Check sheet for the modelled part. Datum: model origin and axes. Units: mm. A direction names the side the tool comes from. Round coordinates to 2 decimals unless told otherwise and drop trailing zeros. Order: outer loops, then holes, each group sorted by start corner. A loop starts at its lowest first (then second) coordinate and runs counter-clockwise, first axis right, second up. Notation, with made-up numbers: (-8.75, 43.25) -> (2.25, 43.25) arc R20 cw to (2.25, 62.25) -> close; hole circle Ø8 at (26.5, -15.5). An arc over 180 degrees is marked (long way). Answer in a Markdown table with one row per item.
```python
from build123d import *

# Parameters (mm, degrees)
SKETCH1_W           = 42
SKETCH1_H           = 42
BOSS_EXTRUDE1_DEPTH = 10.95
CUT_EXTRUDE1_REACH  = 38.9
FILLET1_R           = 2
CUT_EXTRUDE2_DEPTH  = 21.9


with BuildPart() as part:
    # Sketch1 → Boss-Extrude1 (new, symmetric)
    with BuildSketch(Plane.XY):
        Rectangle(SKETCH1_W, SKETCH1_H)
    extrude(amount=BOSS_EXTRUDE1_DEPTH, both=True)

    # Sketch2 → Cut-Extrude1 (cut, up to next)
    with BuildSketch(Plane.XY.offset(10.95), mode=Mode.PRIVATE) as cut_extrude1_sk1:
        Polygon((-21, 21), (-21, 14), (-14, 21), align=None)
    cut_extrude1_tool1 = extrude(cut_extrude1_sk1.sketch, amount=-CUT_EXTRUDE1_REACH, mode=Mode.PRIVATE) & part.part
    # Sketch2 → Cut-Extrude1 (cut, up to next)
    with BuildSketch(Plane.XY.offset(10.95), mode=Mode.PRIVATE) as cut_extrude1_sk2:
        Polygon((-21, -14), (-14, -21), (-21, -21), align=None)
    cut_extrude1_tool2 = extrude(cut_extrude1_sk2.sketch, amount=-CUT_EXTRUDE1_REACH, mode=Mode.PRIVATE) & part.part
    # Sketch2 → Cut-Extrude1 (cut, up to next)
    with BuildSketch(Plane.XY.offset(10.95), mode=Mode.PRIVATE) as cut_extrude1_sk3:
        Polygon((21, -21), (21, -14), (14, -21), align=None)
    cut_extrude1_tool3 = extrude(cut_extrude1_sk3.sketch, amount=-CUT_EXTRUDE1_REACH, mode=Mode.PRIVATE) & part.part
    # Sketch2 → Cut-Extrude1 (cut, up to next)
    with BuildSketch(Plane.XY.offset(10.95), mode=Mode.PRIVATE) as cut_extrude1_sk4:
        Polygon((21, 14), (14, 21), (21, 21), align=None)
    cut_extrude1_tool4 = extrude(cut_extrude1_sk4.sketch, amount=-CUT_EXTRUDE1_REACH, mode=Mode.PRIVATE) & part.part
    add(cut_extrude1_tool1.solids().sort_by_distance((-18.666667, 18.666667, 10.95))[0], mode=Mode.SUBTRACT)
    add(cut_extrude1_tool2.solids().sort_by_distance((-18.666667, -18.666667, 10.95))[0], mode=Mode.SUBTRACT)
    add(cut_extrude1_tool3.solids().sort_by_distance((18.666667, -18.666667, 10.95))[0], mode=Mode.SUBTRACT)
    add(cut_extrude1_tool4.solids().sort_by_distance((18.666667, 18.666667, 10.95))[0], mode=Mode.SUBTRACT)

    # Fillet1
    fillet1_edges = [part.edges().sort_by_distance(p)[0] for p in [
        (21, 14, 0),
        (14, 21, 0),
        (14, -21, 0),
        (21, -14, 0),
        (-21, -14, 0),
        (-14, -21, 0),
        (-14, 21, 0),
        (-21, 14, 0),
    ]]
    fillet(fillet1_edges, radius=FILLET1_R)

    # 3DSketch1 → Cut-Extrude2 (cut)
    with BuildSketch(Plane(origin=(12.757359313, -18, 10.95), x_dir=(-0.5782394408510358, 0.8158671148197367, 0), z_dir=(0, 0, 1))):
        Polygon((0, 0), (1.245796512, -7.308799751), (22.062416383, -22.062416383), (29.371216134, -20.816619871), (44.124832765, 0), (42.879036253, 7.308799751), (22.062416383, 22.062416383), (14.753616632, 20.816619871), align=None)
    extrude(amount=-CUT_EXTRUDE2_DEPTH, mode=Mode.SUBTRACT)


solid = part.part
```
(1) Tool access check on faces 1 (the flat face through (0, 19, 10.95)), 2 (the flat face through (-18, 0, 0)). Record the directions out of +Z, -Z, +X, -X, +Y, -Y that give a thin tool (end or side, any length) a straight path to the whole face; none if there is none.
Solutions:
| item | result |
|---|---|
| face 1 | +Z, +X, -X, +Y, -Y |
| face 2 | +Z, -Z |
(2) Scan lines: probe 1 along X at (y, z) = (12.5, 0); probe 2 along X at (y, z) = (16, 0.25). Record each from-to range of solid material in increasing order. Write a range as from..to.
Solutions:
| item | result |
|---|---|
| probe 1 | -21..-18, 18..21 |
| probe 2 | -19..-14.76, 14.76..19 |
(3) Depth check by flat-ended pin: pin 1 Ø4 at (x, y) = (-15, -2) entering from +Z. Enter the tip coordinate at first touch or a pass-through.
Solutions:
| item | result |
|---|---|
| pin 1 | through |
(4) Section check C-C on z = -2.25. Record the boundary of the cut face in (x, y).
Solutions:
| item | result |
|---|---|
| outline | (-21, -13.17) arc R2 ccw to (-20.41, -14.59) -> (-14.59, -20.41) arc R2 ccw to (-13.17, -21) -> (13.17, -21) arc R2 ccw to (14.59, -20.41) -> (20.41, -14.59) arc R2 ccw to (21, -13.17) -> (21, 13.17) arc R2 ccw to (20.41, 14.59) -> (14.59, 20.41) arc R2 ccw to (13.17, 21) -> (-13.17, 21) arc R2 ccw to (-14.59, 20.41) -> (-20.41, 14.59) arc R2 ccw to (-21, 13.17) -> close; hole (-18, -12.76) -> (-12.76, -18) -> (12.76, -18) -> (18, -12.76) -> (18, 12.76) -> (12.76, 18) -> (-12.76, 18) -> (-18, 12.76) -> close |
(5) Section check A-A on y = -3. Record the boundary of the cut face in (x, z).
Solutions:
| item | result |
|---|---|
| outline | (-21, -10.95) -> (-18, -10.95) -> (-18, 10.95) -> (-21, 10.95) -> close; (18, -10.95) -> (21, -10.95) -> (21, 10.95) -> (18, 10.95) -> close |
(6) Draft check along Y on faces 3 (the flat face through (18, -17, 0)), 4 (the flat face through (15.34, -15.42, 0.15)), 5 (the flat face through (18, 17, 0)). Enter one of: pulls with the +Y half, pulls with the -Y half, needs draft (parallel to the pull), parting line crosses it, or undercut.
Solutions:
| item | result |
|---|---|
| face 3 | pulls with the -Y half |
| face 4 | undercut |
| face 5 | pulls with the +Y half |
